Geometry check sheet. Reference: the model listing, model coordinates, mm. A direction names the side the tool comes from. Coordinates: 2 decimals unless noted, no trailing zeros. Write each loop counter-clockwise with the first axis right and the second up, starting at its lowest first coordinate (ties: lowest second). Pieces come first, ordered by that corner, then holes. Notation, with made-up numbers: (73.5, 89.5) -> (77.5, 89.5) arc R17 ccw to (77.5, 104.5) -> close; hole circle Ø3 at (78, 9.25). An arc over 180 degrees is marked (long way). Answer in a Markdown table with one row per item. Add a question column.
Q1. Section check A-A, the plane x = 21. Record the boundary of the cut face in (y, z).
Q2. Thickness scan on line 1 (Y direction, x = 10, z = 4.5); line 2 (X direction, y = 32, z = 6.25); line 3 (Y direction, x = 31.5, z = -3.75). Record the ranges inside material, lowest first.
Q3. Tool access check on faces 1 (the face through (0.9, 104.14, -4.79)), 2 (the face through (13, 50, 5)), 3 (the face through (45, 49, -10)). Record the directions out of +Z, -Z, +X, -X, +Y, -Y that give a thin tool (end or side, any length) a straight path to the whole face; none if there is none.
Q4. Section check D-D, the plane y = 10. Record the boundary of the cut face in (x, z), and give its area (3 significant figures).
Q5. Release check for a two-part mould opening along Z. For faces 4 (the face through (47.46, 8.09, -9.01)), 5 (the face through (49.14, -4.1, -3.69)), 6 (the face through (23.83, 104.14, -19.1)) record: pulls with the +Z half, pulls with the -Z half, needs draft (parallel to the pull), parting line crosses it, or undercut.
Q6. Gauge pin test, flat ends, axial feed: P1, Ø12, axis at y = 6.5, z = -14.5, coming from the -X side; P2, Ø4, axis at x = 38, y = 7, coming from the -Z side. Record the tip position at first contact, or that the pin passes through.
Q7. Section check B-B, the plane z = -10. Record the boundary of the cut face in (x, y), and give its area (3 significant figures).
Q8. Section check C-C, the plane y = 49. Record the boundary of the cut face in (x, z).
```python
from build123d import *

# Parameters (mm, degrees)
SKIZZE1_W                       = 19
SKIZZE1_H                       = 60
SKIZZE1_R                       = 2.15
AUFSATZ_LINEAR_AUSTRAGEN2_DEPTH = 10
SKIZZE3_W                       = 45
SKIZZE3_H                       = 5
AUFSATZ_LINEAR_AUSTRAGEN3_DEPTH = 20
SKIZZE4_R                       = 2.15
SCHNITT_LINEAR_AUSTRAGEN1_DEPTH = 20
SKIZZE5_R                       = 2.15
SCHNITT_LINEAR_AUSTRAGEN2_DEPTH = 120
VERRUNDUNG1_R                   = 3


with BuildPart() as part:
    # Skizze1 → Aufsatz-Linear austragen2 (new body)
    with BuildSketch(Plane.XY):
        Polygon((0, -5), (50, -5), (50, 105), (0, 105), (0, 90), (0, 10), align=None)
        with Locations((22.5, 50)):
            Rectangle(SKIZZE1_W, SKIZZE1_H, mode=Mode.SUBTRACT)
        with Locations((35, 10)):
            Circle(SKIZZE1_R, mode=Mode.SUBTRACT)
        with Locations((10, 10)):
            Circle(SKIZZE1_R, mode=Mode.SUBTRACT)
        with Locations((35, 90)):
            Circle(SKIZZE1_R, mode=Mode.SUBTRACT)
        with Locations((10, 90)):
            Circle(SKIZZE1_R, mode=Mode.SUBTRACT)
    extrude(amount=AUFSATZ_LINEAR_AUSTRAGEN2_DEPTH)

    # Skizze3 → Aufsatz-Linear austragen3 (add)
    with BuildSketch(Plane(origin=(0, 0, 0), x_dir=(-1, 0, 0), z_dir=(0, 0, -1))):
        Polygon((-45, 105), (-50, 105), (-50, -5), (-45, -5), (-45, 0), (-45, 100), align=None)
        with Locations((-22.5, 102.5)):
            Rectangle(SKIZZE3_W, SKIZZE3_H)
        with Locations((-22.5, -2.5)):
            Rectangle(SKIZZE3_W, SKIZZE3_H)
    extrude(amount=AUFSATZ_LINEAR_AUSTRAGEN3_DEPTH)

    # Skizze4 → Schnitt-Linear austragen1 (cut)
    with BuildSketch(Plane.ZY.offset(-45)):
        with Locations((-10, 90)):
            Circle(SKIZZE4_R)
        with Locations((-10, 10)):
            Circle(SKIZZE4_R)
    extrude(amount=-SCHNITT_LINEAR_AUSTRAGEN1_DEPTH, mode=Mode.SUBTRACT)

    # Skizze5 → Schnitt-Linear austragen2 (cut)
    with BuildSketch(Plane(origin=(0, 105, 0), x_dir=(1, 0, 0), z_dir=(0, 1, 0))):
        with Locations((10, 10)):
            Circle(SKIZZE5_R)
    extrude(amount=-SCHNITT_LINEAR_AUSTRAGEN2_DEPTH, mode=Mode.SUBTRACT)

    # Verrundung1
    verrundung1_edges = [part.edges().sort_by_distance(p)[0] for p in [
        (50, 105, -5),
        (50, -5, -5),
        (0, -5, -5),
        (0, 105, -5),
        (25, 105, -20),
        (50, 50, -20),
        (25, -5, -20),
    ]]
    fillet(verrundung1_edges, radius=VERRUNDUNG1_R)


solid = part.part
```
Calculated:
| question | item | result |
|---|---|---|
| 1 | outline | (-5, -17) arc R3 ccw to (-2, -20) -> (0, -20) -> (0, 0) -> (20, 0) -> (20, 10) -> (-5, 10) -> close; (80, 0) -> (100, 0) -> (100, -20) -> (102, -20) arc R3 ccw to (105, -17) -> (105, 10) -> (80, 10) -> close |
| 2 | line 1 | y = -5 to 7.85, 12.15 to 87.85, 92.15 to 105 |
| 2 | line 2 | x = 0 to 13, 32 to 50 |
| 2 | line 3 | y = -5 to 0, 100 to 105 |
| 3 | face 1 | +Z, -Z, -X, +Y |
| 3 | face 2 | +Z, -Z |
| 3 | face 3 | -Z, -X |
| 4 | outline | (0, 0) -> (7.85, 0) -> (7.85, 10) -> (0, 10) -> close; (12.15, 0) -> (32.85, 0) -> (32.85, 10) -> (12.15, 10) -> close; (37.15, 0) -> (45, 0) -> (45, -7.85) -> (50, -7.85) -> (50, 10) -> (37.15, 10) -> close; (45, -20) -> (47, -20) arc R3 ccw to (50, -17) -> (50, -12.15) -> (45, -12.15) -> close |
| 4 | area | 491 mm² |
| 5 | face 4 | undercut |
| 5 | face 5 | needs draft |
| 5 | face 6 | pulls with the -Z half |
| 6 | P1 | stops at x = 45 |
| 6 | P2 | stops at z = 0 |
| 7 | outline | (0, -2) arc R3 ccw to (3, -5) -> (7.85, -5) -> (7.85, 0) -> (0, 0) -> close; (0, 100) -> (7.85, 100) -> (7.85, 105) -> (3, 105) arc R3 ccw to (0, 102) -> close; (12.15, -5) -> (47, -5) arc R3 ccw to (50, -2) -> (50, 7.85) -> (45, 7.85) -> (45, 0) -> (12.15, 0) -> close; (12.15, 100) -> (45, 100) -> (45, 92.15) -> (50, 92.15) -> (50, 102) arc R3 ccw to (47, 105) -> (12.15, 105) -> close; (45, 12.15) -> (50, 12.15) -> (50, 87.85) -> (45, 87.85) -> close |
| 7 | area | 906 mm² |
| 8 | outline | (0, 0) -> (13, 0) -> (13, 10) -> (0, 10) -> close; (32, 0) -> (45, 0) -> (45, -20) -> (47, -20) arc R3 ccw to (50, -17) -> (50, 10) -> (32, 10) -> close |
